Geometry: final body of the model. Coordinates: model frame, mm. Face numbers are marked on the shaded views. A direction names the side the tool comes from. Give positions to 0.01 mm unless a question says otherwise; leave off trailing zeros. Order: outer loops, then holes, each group sorted by start corner. A loop starts at its lowest first (then second) coordinate and runs counter-clockwise, first axis right, second up. Notation, with made-up numbers: M 73,14 L 93,14 A21 ccw 93,33 Z; hole C 78.25,89.25 d8. An arc over 180 degrees is marked long. Use CSV: the item, a comma, the result in double quotes.
Autodesk Inventor part; units mm, degrees
ref_plane "YZ Plane" through (0, 0, 0) normal (1, 0, 0) x (0, 1, 0)
ref_plane "XZ Plane" through (0, 0, 0) normal (0, 1, 0) x (-1, 0, 0)
ref_plane "XY Plane" through (0, 0, 0) normal (0, 0, 1) x (1, 0, 0)
sketch "Skizze1" plane through (0, 0, 0) normal (0, 0, 1) x (1, 0, 0)
  line L0 (0, 7) -> (0, -7) construction
  line L1 (-10.5, 0) -> (28, 0) construction
  circle A0 centre (0, 0) radius 2
  circle A1 centre (13, 0) radius 1.3257
  circle A2 centre (17, 0) radius 1.3
  circle A3 centre (20, 0) radius 1.3
  arc A4 (20.3125, -2.4804) -> (20.3125, 2.4804) centre (20, 0) ccw
  arc A5 (0.625, 4.9608) -> (0.625, -4.9608) centre (0, 0) ccw
  line L2 (0.625, 4.9608) -> (20.3125, 2.4804)
  line L3 (0.625, -4.9608) -> (20.3125, -2.4804)
  line L4 (0.625, -4.9608) -> (0.625, -1.8998)
  line L5 (0.625, 1.8998) -> (0.625, 4.9608)
  line L6 (0.625, 1.8998) -> (0.625, -1.8998)
  dimension "d0" = 13
  dimension "d1" = 17
  dimension "d2" = 20
  dimension "d3" = 5
  dimension "d4" = 2.6
  dimension "d5" = 4
  dimension "d6" = 10
extrude "Extrusion1" add sketch "Skizze1" along normal blind 3
extrude "Extrusion2" add sketch "Skizze1" along normal blind 5 contours L6 A0 | A0 L4 A5 L5 picked at (-0.25, 0)
chamfer "Fase1" distance 10 distance2 2 1 edges at (0.625, 0, 3) measured on face at (4.3081, 0, 3)
extrude "Extrusion3" cut sketch "Skizze1" along normal blind 5 contours A0 L6 | L6 A0
properties part number "Servo-Arm-20mm"
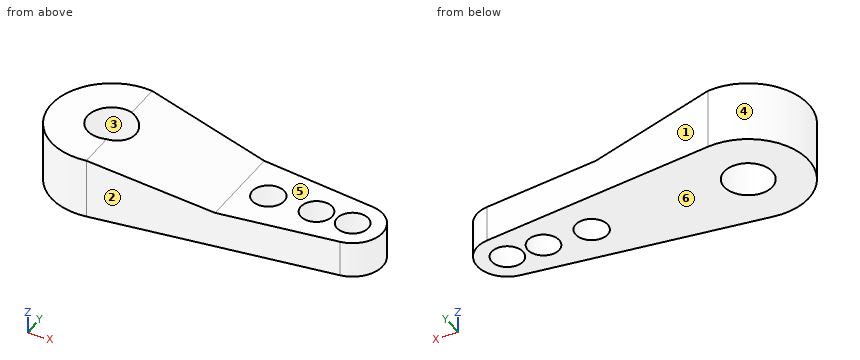
1. Line query: line 1 (Y direction, x = 0, z = 3.5); line 2 (X direction, y = -0.5, z = 1.25); line 3 (Y direction, x = 17, z = 0.9). Output: solid intervals per line, ascending.
Answer:
line 1,"-5 to -2, 2 to 5"
line 2,"-4.97 to -1.94, 1.94 to 11.77, 14.23 to 15.8, 18.2 to 18.8, 21.2 to 22.45"
line 3,"-2.9 to -1.3, 1.3 to 2.9"
2. Reachability of the marked faces 5 and 6 from +Z, -Z, +X, -X, +Y, -Y: full face, straight path, thin tool, end or side. Return the list, or none.
Answer:
face 5,"+Z, +X, +Y, -Y"
face 6,"-Z, +X, -X, +Y, -Y"
3. Section A-A, the plane x = 0. Return the cut outline in (y, z), plus the area to 3 significant figures.
Answer:
outline,"M -5,0 L -2,0 L -2,5 L -5,5 Z; M 2,0 L 5,0 L 5,5 L 2,5 Z"
area,"30.0 mm2"
4. Section B-B, the plane y = 0. Return the cut outline in (x, z), plus the area to 3 significant figures.
Answer:
outline,"M -5,0 L -2,0 L -2,5 L -5,5 Z; M 2,0 L 11.67,0 L 11.67,3 L 10.62,3 L 2,4.72 Z; M 14.33,0 L 15.7,0 L 15.7,3 L 14.33,3 Z; M 18.3,0 L 18.7,0 L 18.7,3 L 18.3,3 Z; M 21.3,0 L 22.5,0 L 22.5,3 L 21.3,3 Z"
area,"60.4 mm2"
5. Pin query (flat end, axial travel): pin 1 Ø2 at (x, y) = (15, -1) entering from +Z; pin 2 Ø5 at (x, y) = (7, -2.5) entering from -Z; pin 3 Ø3 at (x, z) = (18, 0.5) entering from -Y. Return the tip coordinate at first contact, or that it passes through.
Answer:
pin 1,"z = 3"
pin 2,"z = 0"
pin 3,"y = -2.96"
6. Section D-D, the plane x = 13. Return the cut outline in (y, z), plus the area to 3 significant figures.
Answer:
outline,"M -3.4,0 L -1.33,0 L -1.33,3 L -3.4,3 Z; M 1.33,0 L 3.4,0 L 3.4,3 L 1.33,3 Z"
area,"12.5 mm2"
7. Pull-direction query (Y, two-part tool) for the marked faces 1, 2, 3 and 4; classes: +Y half, -Y half, draft (parallel to the pull), parting line (faces both ways), or undercut.
Answer:
face 1,"+Y half"
face 2,"-Y half"
face 3,"undercut"
face 4,"parting line"
